```python
from build123d import *

# Parameters (mm, degrees)
F0_W     = 1
F0_H     = 1
F1_DEPTH = 9
F2_W     = 1
F2_H     = 1
F3_DEPTH = 1
F4_W     = 1
F4_H     = 1
F5_DEPTH = 1


with BuildPart() as f1:
    # F0 (on Front) → F1 (new body)
    with BuildSketch(Plane.XZ):
        Polygon((-9, 1), (-16, 1), (-16, 0), (16, 0), (16, 1), (9, 1), (8, 1), (-8, 1), align=None)
        with Locations((-8.5, 1.5)):
            Rectangle(F0_W, F0_H)
        with Locations((8.5, 1.5)):
            Rectangle(F0_W, F0_H)
    extrude(amount=F1_DEPTH)

    # F2 (on face) → F3 (cut)
    with BuildSketch(Plane.XZ.offset(9)):
        Polygon((-9.9123697728, 3.1492931303), (-9.9123697728, 1), (-9, 1), (-9, 2), (-8, 2), (-8, 1), (8, 1), (8, 2), (9, 2), (9, 1), (10.0291045383, 1), (10.0291045383, 3.1492931303), align=None)
        with Locations((-8.5, 1.5)):
            Rectangle(F2_W, F2_H)
        with Locations((8.5, 1.5)):
            Rectangle(F2_W, F2_H)
    extrude(amount=-F3_DEPTH, mode=Mode.SUBTRACT)

    # F4 (on face) → F5 (cut)
    with BuildSketch(Plane(origin=(0, 0, 0), x_dir=(-1, 0, 0), z_dir=(0, 1, 0))):
        with Locations((-8.5, 1.5)):
            Rectangle(F4_W, F4_H)
        with Locations((8.5, 1.5)):
            Rectangle(F4_W, F4_H)
    extrude(amount=-F5_DEPTH, mode=Mode.SUBTRACT)


solid = f1.part
```
Geometry: final body of the model. Coordinates: model frame, mm. A direction names the side the tool comes from. Round coordinates to 2 decimals unless told otherwise and drop trailing zeros. Order: outer loops, then holes, each group sorted by start corner. A loop starts at its lowest first (then second) coordinate and runs counter-clockwise, first axis right, second up. Notation, with made-up numbers: (24, 82) - (45, 82) arc R32 ccw to (45, 109) - close; hole circle Ø3 at (-20.75, -7.75). An arc over 180 degrees is marked (long way). Write item = value, one per line. Start each with the question number.
Q1. Cut plane C-C on x = 1. Return the cut outline in (y, z).
Q2. Access query for faces 1 (the flat face through (8.5, -8, 1.5)), 2 (the flat face through (9, -4.5, 1.5)), 3 (the flat face through (-8.5, -1, 1.5)), 4 (the flat face through (-9, -4.5, 1.5)), 5 (the flat face through (-8, -4.5, 1.5)). Directions: +Z, -Z, +X, -X, +Y, -Y. A direction counts if a zero-diameter tool reaches every point of the face in a straight line with its end or side. Return the directions, or none.
Q3. Cut plane B-B on y = -2.5. Return the cut outline in (x, z), and give its area (3 significant figures).
Q4. Cut plane D-D on y = -0.5. Return the cut outline in (x, z), and give its area (3 significant figures).
Q5. Pin query (flat end, axial travel): pin 1 (0.8 mm diameter, centred on x = 8.5, z = 1.5, fed in from -Y); pin 2 (0.8 mm diameter, centred on y = -4.5, z = 1.5, fed in from -X); pin 3 (0.8 mm diameter, centred on x = 8.5, z = 1.5, fed in from +Y). Return the tip coordinate at first contact, or that it passes through.
Q6. Cut plane A-A on z = 1.3. Return the cut outline in (x, y), and give its area (3 significant figures).
Q7. Ray query, line 1 (X direction, y = -6.5, z = 1.2); line 2 (Z direction, x = 9.5, y = -8.25). Return the intervals inside material, ascending. Write a range as from..to.
Outcome:
q1.outline = (-9, 0) - (0, 0) - (0, 1) - (-9, 1) - close
q2.face_1 = +Z, +X, -X, -Y
q2.face_2 = +Z, +X, +Y, -Y
q2.face_3 = +Z, +X, -X, +Y
q2.face_4 = +Z, -X, +Y, -Y
q2.face_5 = +Z, +Y, -Y
q3.outline = (-16, 0) - (16, 0) - (16, 1) - (9, 1) - (9, 2) - (8, 2) - (8, 1) - (-8, 1) - (-8, 2) - (-9, 2) - (-9, 1) - (-16, 1) - close
q3.area = 34.0 mm^2
q4.outline = (-16, 0) - (16, 0) - (16, 1) - (-16, 1) - close
q4.area = 32.0 mm^2
q5.pin_1 = -8
q5.pin_2 = -9
q5.pin_3 = -1
q6.outline = (-9, -8) - (-8, -8) - (-8, -1) - (-9, -1) - close; (8, -8) - (9, -8) - (9, -1) - (8, -1) - close
q6.area = 14.0 mm^2
q7.line_1 = -9..-8, 8..9
q7.line_2 = 0..1
